from build123d import *

# Parameters (mm, degrees)
SKETCH1_R           = 2.5
BOSS_EXTRUDE1_DEPTH = 100


with BuildPart() as part:
    # Sketch1 → Boss-Extrude1 (new body)
    with BuildSketch(Plane.XY):
        with BuildLine():
            Line((1.971572875, 3.9), (-1.971572875, 3.9))
            ThreePointArc((-1.971572875, 3.9), (-2.73693974, 4.052240935), (-3.385786438, 4.485786438))
            Line((-3.385786438, 4.485786438), (-5.5, 6.6))
            Line((-5.5, 6.6), (-5.5, 8.2))
            Line((-5.5, 8.2), (-3.6, 8.2))
            Line((-3.6, 8.2), (-3.6, 8.5))
            Line((-3.6, 8.5), (-3.1, 8.5))
            Line((-3.1, 8.5), (-3.1, 10))
            Line((-3.1, 10), (-8.5, 10))
            ThreePointArc((-8.5, 10), (-9.560660172, 9.560660172), (-10, 8.5))
            Line((-10, 8.5), (-10, 3.1))
            Line((-10, 3.1), (-8.5, 3.1))
            Line((-8.5, 3.1), (-8.5, 3.6))
            Line((-8.5, 3.6), (-8.2, 3.6))
            Line((-8.2, 3.6), (-8.2, 5.5))
            Line((-8.2, 5.5), (-6.6, 5.5))
            Line((-6.6, 5.5), (-4.485786438, 3.385786438))
            ThreePointArc((-4.485786438, 3.385786438), (-4.052240935, 2.73693974), (-3.9, 1.971572875))
            Line((-3.9, 1.971572875), (-3.9, -1.971572875))
            ThreePointArc((-3.9, -1.971572875), (-4.052240935, -2.73693974), (-4.485786438, -3.385786438))
            Line((-4.485786438, -3.385786438), (-6.6, -5.5))
            Line((-6.6, -5.5), (-8.2, -5.5))
            Line((-8.2, -5.5), (-8.2, -3.6))
            Line((-8.2, -3.6), (-8.5, -3.6))
            Line((-8.5, -3.6), (-8.5, -3.1))
            Line((-8.5, -3.1), (-10, -3.1))
            Line((-10, -3.1), (-10, -8.5))
            ThreePointArc((-10, -8.5), (-9.560660172, -9.560660172), (-8.5, -10))
            Line((-8.5, -10), (-3.1, -10))
            Line((-3.1, -10), (-3.1, -8.5))
            Line((-3.1, -8.5), (-3.6, -8.5))
            Line((-3.6, -8.5), (-3.6, -8.2))
            Line((-3.6, -8.2), (-5.5, -8.2))
            Line((-5.5, -8.2), (-5.5, -6.6))
            Line((-5.5, -6.6), (-3.385786438, -4.485786438))
            ThreePointArc((-3.385786438, -4.485786438), (-2.73693974, -4.052240935), (-1.971572875, -3.9))
            Line((-1.971572875, -3.9), (1.971572875, -3.9))
            ThreePointArc((1.971572875, -3.9), (2.73693974, -4.052240935), (3.385786438, -4.485786438))
            Line((3.385786438, -4.485786438), (5.5, -6.6))
            Line((5.5, -6.6), (5.5, -8.2))
            Line((5.5, -8.2), (3.6, -8.2))
            Line((3.6, -8.2), (3.6, -8.5))
            Line((3.6, -8.5), (3.1, -8.5))
            Line((3.1, -8.5), (3.1, -10))
            Line((3.1, -10), (8.5, -10))
            ThreePointArc((8.5, -10), (9.560660172, -9.560660172), (10, -8.5))
            Line((10, -8.5), (10, -3.1))
            Line((10, -3.1), (8.5, -3.1))
            Line((8.5, -3.1), (8.5, -3.6))
            Line((8.5, -3.6), (8.2, -3.6))
            Line((8.2, -3.6), (8.2, -5.5))
            Line((8.2, -5.5), (6.6, -5.5))
            Line((6.6, -5.5), (4.485786438, -3.385786438))
            ThreePointArc((4.485786438, -3.385786438), (4.052240935, -2.73693974), (3.9, -1.971572875))
            Line((3.9, -1.971572875), (3.9, 1.971572875))
            ThreePointArc((3.9, 1.971572875), (4.052240935, 2.73693974), (4.485786438, 3.385786438))
            Line((4.485786438, 3.385786438), (6.6, 5.5))
            Line((6.6, 5.5), (8.2, 5.5))
            Line((8.2, 5.5), (8.2, 3.6))
            Line((8.2, 3.6), (8.5, 3.6))
            Line((8.5, 3.6), (8.5, 3.1))
            Line((8.5, 3.1), (10, 3.1))
            Line((10, 3.1), (10, 8.5))
            ThreePointArc((10, 8.5), (9.560660172, 9.560660172), (8.5, 10))
            Line((8.5, 10), (3.1, 10))
            Line((3.1, 10), (3.1, 8.5))
            Line((3.1, 8.5), (3.6, 8.5))
            Line((3.6, 8.5), (3.6, 8.2))
            Line((3.6, 8.2), (5.5, 8.2))
            Line((5.5, 8.2), (5.5, 6.6))
            Line((5.5, 6.6), (3.385786438, 4.485786438))
            ThreePointArc((3.385786438, 4.485786438), (2.73693974, 4.052240935), (1.971572875, 3.9))
        make_face()
        Circle(SKETCH1_R, mode=Mode.SUBTRACT)
    extrude(amount=BOSS_EXTRUDE1_DEPTH)


solid = part.part
For this review, take the finished solid that the model builds, in its own axes (mm). A direction names the side the tool comes from. Give positions to 0.01 mm unless a question says otherwise; leave off trailing zeros. Loops run counter-clockwise (first coordinate to the right, second up) from the corner with the lowest first, then second, coordinate; pieces in that order, holes last. Notation, with made-up numbers: M -15,-11.5 L -5,-11.5 A6 cw -5,-5.5 Z; hole C 83,-3.75 d4. An arc over 180 degrees is marked long. Answer as a JSON object with one key per item and string values. Group by question number.
Q1. Insertion check: P1, Ø3, axis at x = 0, z = 55, coming from the +Y side; P2, Ø1.5, axis at x = 0.5, z = 28.5, coming from the -Y side; P3, Ø1.5, axis at x = 0.5, y = 5, coming from the -Z side (3 decimals). Each pin has a flat end and moves straight along its axis. Give the tip position at first contact, or say it passes through.
Q2. For probe 1 along Y at (x, z) = (-6.75, 8); probe 2 along X at (y, z) = (-3.75, 94), list the stretches that pass through material, from the lowest coordinate up. Write a range as [from, to].
Q3. Tool access review of faces 1 (the flat face through (-3.9, 0, 49)), 2 (the flat face through (0, 3.9, 49)), 3 (the flat face through (3.9, 0, 49)), 4 (the flat face through (-5, 8.2, 49)): name each direction out of +Z, -Z, +X, -X, +Y, -Y from which nothing blocks a thin tool from reaching the whole face with its end or side.
Q4. Add section A-A on y = 0. Give the boundary of the cut face in (x, z).
Q5. Mouldability with a two-part tool opening along Y and no side actions: class faces 5 (the flat face through (6, 10, 49)), 6 (the flat face through (-7, -5.5, 49)), 7 (the flat face through (10, -6, 49)) as +Y half, -Y half, draft (parallel to the pull), parting line (faces both ways), or undercut.
Checked values:
{
 "1": {"P1": "y = 3.9", "P2": "y = -3.9", "P3": "through"},
 "2": {"probe 1": "[-10, -5.5], [5.5, 10]", "probe 2": "[-10, -8.2], [-4.85, 4.85], [8.2, 10]"},
 "3": {"face 1": "+Z, -Z, -X", "face 2": "+Z, -Z, +Y", "face 3": "+Z, -Z, +X", "face 4": "+Z, -Z"},
 "4": {"outline": "M -3.9,0 L -2.5,0 L -2.5,100 L -3.9,100 Z; M 2.5,0 L 3.9,0 L 3.9,100 L 2.5,100 Z"},
 "5": {"face 5": "+Y half", "face 6": "undercut", "face 7": "draft"}
}
